from build123d import *

# Parameters (mm, degrees)
BOSS_EXTRU_7_DEPTH      = 35
BOSS_EXTRU_8_START      = -5
BOSS_EXTRU_8_DEPTH      = 5
ESQUISSE3_R             = 2.4999999999999987
ENL_V_MAT_EXTRU_1_DEPTH = 5
ENL_V_MAT_EXTRU_2_DEPTH = 12
ESQUISSE6_R             = 9.75
ENL_V_MAT_EXTRU_3_DEPTH = 5


with BuildPart() as part:
    # Esquisse1 → Boss.-Extru.7 (new, symmetric)
    with BuildSketch(Plane(origin=(0, 0, 0), x_dir=(1, 0, 0), z_dir=(0, 1, 0))):
        with BuildLine():
            Line((0, 51.00000000000001), (1.188e-14, 46.00000000000001))
            ThreePointArc((1.188e-14, 46.00000000000001), (-12.921623376513631, 44.33590628857987), (-24.99999999999999, 39.45222154178573))
            Line((-24.99999999999999, 39.45222154178573), (-24.99999999999999, -39.45222154178573))
            ThreePointArc((-24.99999999999999, -39.45222154178573), (-12.921623376513633, -44.33590628857988), (1.188e-14, -46.00000000000001))
            Line((1.188e-14, -46.00000000000001), (0, -51.00000000000001))
            ThreePointArc((0, -51.00000000000001), (-18.830584522511188, -47.39629823668259), (-35, -37.09447398198281))
            Line((-35, -37.09447398198281), (-35, 37.09447398198281))
            ThreePointArc((-35, 37.09447398198281), (-18.830584522511195, 47.396298236682604), (0, 51.00000000000001))
        make_face()
    extrude(amount=BOSS_EXTRU_7_DEPTH, both=True)

    # Esquisse2 → Boss.-Extru.8 (add)
    with BuildSketch(Plane.XZ.offset(35).offset(BOSS_EXTRU_8_START)):
        with BuildLine():
            Line((-34.99999999999999, 37.094473981982816), (-34.99999999999999, -37.094473981982816))
            ThreePointArc((-34.99999999999999, -37.094473981982816), (-18.830584522511195, -47.396298236682604), (0, -51.00000000000001))
            Line((0, -51.00000000000001), (0, 51.00000000000001))
            ThreePointArc((0, 51.00000000000001), (-18.830584522511195, 47.396298236682604), (-34.99999999999999, 37.094473981982816))
        make_face()
    extrude(amount=BOSS_EXTRU_8_DEPTH)

    # Esquisse3 → Enlèv. mat.-Extru.1 (cut)
    with BuildSketch(Plane(origin=(-24.99999999999999, 0, 0), x_dir=(0, 0, -1), z_dir=(1, 0, 0))):
        with Locations((-19.600000000000012, -2.2100000000000035)):
            Circle(ESQUISSE3_R)
        with Locations((19.59999999999999, -2.209999999999999)):
            Circle(ESQUISSE3_R)
    extrude(amount=-ENL_V_MAT_EXTRU_1_DEPTH, mode=Mode.SUBTRACT)

    # Esquisse5 → Enlèv. mat.-Extru.2 (cut)
    with BuildSketch(Plane(origin=(0, 0, 0), x_dir=(2.38e-15, 0, -1), z_dir=(1, 0, 2.38e-15))):
        with BuildLine():
            Line((40.674477228026994, 51.032394682771525), (98.05120693404734, 14.815086571109495))
            ThreePointArc((98.05120693404734, 14.815086571109495), (1.023e-14, -17), (-98.05120693404734, 14.81508657110947))
            Line((-98.05120693404734, 14.81508657110947), (-40.674477228026994, 51.03239468277152))
            ThreePointArc((-40.674477228026994, 51.03239468277152), (6.55e-15, 43.000000000000014), (40.674477228026994, 51.032394682771525))
        make_face()
    extrude(amount=-ENL_V_MAT_EXTRU_2_DEPTH, mode=Mode.SUBTRACT)

    # Esquisse6 → Enlèv. mat.-Extru.3 (cut)
    with BuildSketch(Plane(origin=(-24.99999999999999, 0, 0), x_dir=(0, 0, -1), z_dir=(1, 0, 0))):
        with Locations((0, 20.000000000000004)):
            Circle(ESQUISSE6_R)
    extrude(amount=-ENL_V_MAT_EXTRU_3_DEPTH, mode=Mode.SUBTRACT)


solid = part.part
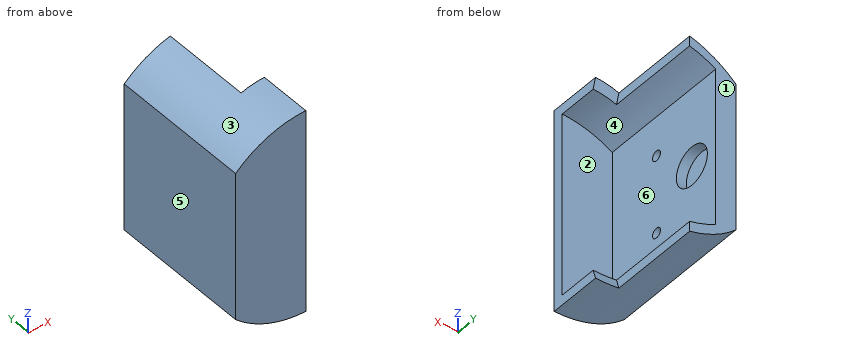
Could you check a few things on this model? Use its own coordinates, in mm. Face numbers are marked on the shaded views. A direction names the side the tool comes from. Coordinates: 2 decimals unless noted, no trailing zeros. Order: outer loops, then holes, each group sorted by start corner. A loop starts at its lowest first (then second) coordinate and runs counter-clockwise, first axis right, second up. Notation, with made-up numbers: (28.25, 29) - (61.25, 29) arc R23 ccw to (61.25, 54) - close; hole circle Ø9 at (83, 37). An arc over 180 degrees is marked (long way). Answer in a Markdown table with one row per item. Add a question column.
(1) If we section it at D-D, the plane x = -14: Please give me the cut outline in (y, z).
(2) Will these pins go through, and if not, where does the flat tip stop? pin 1 (8 mm diameter, centred on y = -2.21, z = -19.6, fed in from +X); pin 2 (1.5 mm diameter, centred on y = 17, z = -46.5, fed in from +X); pin 3 (7.5 mm diameter, centred on x = -14.5, z = 9, fed in from +Y).
(3) I need wall thicknesses on L1, parallel to Y at x = -28.25, z = 19.6; L2, parallel to X at y = -24, z = -10; L3, parallel to Y at x = -3, z = -17.5. Which ranges of each line are inside material? Lowest first, please.
(4) If we section it at C-C, the plane x = -28.5: Please give me the cut outline in (y, z), then the cut area to 3 significant figures.
(5) If we section it at A-A, the plane y = 20: Please give me the cut outline in (x, z), then the cut area to 3 significant figures.
(6) If we mould it in two halves opening along Z, with no side actions, what happens to the marked faces 1, 2, 3 and 4? For each: released by +Z, released by -Z, zero draft, split by the parting line, or undercut.
(7) On a 3-axis mill with a long thin cutter (end or side, diameter ignored), from which of +Z, -Z, +X, -X, +Y, -Y can I reach the whole of each face in a straight line? I mean the marked faces 5 and 6. Say none if no direction works.
(8) If we section it at B-B, the plane z = -35.5: Please give me the cut outline in (x, y), then the cut area to 3 significant figures.
Results are:
| question | item | result |
|---|---|---|
| 1 | outline | (-35, -49.04) - (35, -49.04) - (35, -44.04) - (-30, -44.04) - (-30, 44.04) - (35, 44.04) - (35, 49.04) - (-35, 49.04) - close |
| 2 | pin 1 | stops at x = -25 |
| 2 | pin 2 | stops at x = -12 |
| 2 | pin 3 | stops at y = -30 |
| 3 | L1 | y = -35 to -4.71, 0.29 to 35 |
| 3 | L2 | x = -35 to -25 |
| 3 | L3 | y = -35 to -30 |
| 4 | outline | (-35, -42.29) - (35, -42.29) - (35, 42.29) - (-35, 42.29) - close; hole circle Ø5 at (-2.21, -19.6); hole circle Ø5 at (-2.21, 19.6); hole circle Ø19.5 at (20, 0) |
| 4 | area | 5,580 mm2 |
| 5 | outline | (-35, -37.09) arc R51 ccw to (-12, -49.57) - (-12, -44.57) arc R51 cw to (-25, -39.45) - (-25, -9.75) - (-30, -9.75) - (-30, 9.75) - (-25, 9.75) - (-25, 39.45) arc R51 cw to (-12, 44.57) - (-12, 49.57) arc R51 ccw to (-35, 37.09) - close |
| 5 | area | 854 mm2 |
| 6 | face 1 | zero draft |
| 6 | face 2 | undercut |
| 6 | face 3 | released by +Z |
| 6 | face 4 | undercut |
| 7 | face 5 | +Z, -Z, -X, +Y, -Y |
| 7 | face 6 | +X, +Y |
| 8 | outline | (-35, -35) - (0, -35) - (0, -30) - (-25, -30) - (-25, 35) - (-35, 35) - close |
| 8 | area | 825 mm2 |
